Here's how the part is built. I have some questions about the finished solid (model axes, mm). Face numbers are marked on the shaded views. A direction names the side the tool comes from. Round coordinates to 2 decimals unless told otherwise and drop trailing zeros. Loops run counter-clockwise (first coordinate to the right, second up) from the corner with the lowest first, then second, coordinate; pieces in that order, holes last. Notation, with made-up numbers: (73.5, 27) - (88.5, 27) arc R13 ccw to (88.5, 41) - close; hole circle Ø11 at (-4, 51). An arc over 180 degrees is marked (long way). Answer as a JSON object with one key per item and string values. Group by question number.
1) Which directions (+Z, -Z, +X, -X, +Y, -Y) give clear straight access to the entire face, cutting with the end or side of a thin tool? Please do the marked faces 1, 2 and 3.
2) I want a section at A-A, the plane x = 3. Please give me the cut outline in (y, z).
3) Will these pins go through, and if not, where does the flat tip stop? P1, Ø4, axis at y = 22.5, z = 5.5, coming from the +X side; P2, Ø2, axis at y = 5, z = -2.5, coming from the -X side; P3, Ø3, axis at x = 18, z = -0.5, coming from the +Y side.
4) I want a section at B-B, the plane y = 33. Please give me the cut outline in (x, z), then the cut area to 3 significant figures.
5) If I drill on line 1 along X through (y, z) = (36, -5); line 2 along Y through (x, z) = (21, 5.5); line 3 along Y through (x, z) = (18, 1.75), over which ranges is the centre line in solid material (lowest first)? Write a range as [from, to].
from build123d import *

# Parameters (mm, degrees)
SKETCH_1_W             = 40
SKETCH_1_H             = 20
EXTRUDE_1_DEPTH        = 37
SKETCH_2_W             = 20
SKETCH_2_H             = 2.5
EXTRUDE_2_DEPTH        = 7
FILLET_1_R             = 1
CUT_EXTRUDE_1_DEPTH    = 47
FILLET_1_OF_MIRROR_1_R = 1
EXTRUDE_3_DEPTH        = 2.5
SKETCH_6_R             = 6.5
EXTRUDE_4_DEPTH        = 3.5
SKETCH_7_R             = 5.5
EXTRUDE_5_DEPTH        = 4
SKETCH_8_R             = 3
EXTRUDE_6_DEPTH        = 8
CHAMFER_1_SIZE         = 2


with BuildPart() as part:
    # 草图1 → 凸台-拉伸1 (new body)
    with BuildSketch(Plane(origin=(0, 0, 0), x_dir=(1, 0, 0), z_dir=(0, 1, 0))):
        Rectangle(SKETCH_1_W, SKETCH_1_H)
    extrude(amount=EXTRUDE_1_DEPTH)

    # 草图2 → 凸台-拉伸2 (add)
    with BuildSketch(Plane(origin=(20, 0, 0), x_dir=(0, 0, -1), z_dir=(1, 0, 0))):
        with Locations((0, 28.75)):
            Rectangle(SKETCH_2_W, SKETCH_2_H)
    extrude_2 = extrude(amount=EXTRUDE_2_DEPTH)

    # 圆角1
    fillet_1_edges = [part.edges().sort_by_distance(p)[0] for p in [
        (27, 28.75, -10),
        (27, 28.75, 10),
    ]]
    fillet(fillet_1_edges, radius=FILLET_1_R)

    # 草图3 → 切除-拉伸1 (cut)
    with BuildSketch(Plane(origin=(0, 0, 0), x_dir=(1, 0, 0), z_dir=(0, 1, 0))):
        with BuildLine():
            Line((25.882021082, 5.209730705), (27, 5.209730705))
            Line((27, 5.209730705), (27, 3.27640675))
            Line((27, 3.27640675), (25.792986763, 3.27640675))
            ThreePointArc((25.792986763, 3.27640675), (22.077686149, 4.416217577), (25.882021082, 5.209730705))
        make_face()
        with BuildLine():
            Line((27, -3.27640675), (25.792986763, -3.27640675))
            ThreePointArc((25.792986763, -3.27640675), (22.077686149, -4.416217577), (25.882021082, -5.209730705))
            Line((25.882021082, -5.209730705), (27, -5.209730705))
            Line((27, -5.209730705), (27, -3.27640675))
        make_face()
    cut_extrude_1 = extrude(amount=CUT_EXTRUDE_1_DEPTH, mode=Mode.SUBTRACT)

    # 镜向1: 凸台-拉伸2, 切除-拉伸1 across plane
    add(extrude_2.mirror(Plane(origin=(0, 0, 0), x_dir=(0, 0, 1), z_dir=(1, 0, 0))))
    add(cut_extrude_1.mirror(Plane(origin=(0, 0, 0), x_dir=(0, 0, 1), z_dir=(1, 0, 0))), mode=Mode.SUBTRACT)

    # 圆角1 of 镜向1
    fillet_1_of_mirror_1_edges = [part.edges().sort_by_distance(p)[0] for p in [
        (-27, 28.75, -10),
        (-27, 28.75, 10),
    ]]
    fillet(fillet_1_of_mirror_1_edges, radius=FILLET_1_OF_MIRROR_1_R)

    # 草图4 → 凸台-拉伸3 (add)
    with BuildSketch(Plane(origin=(0, 37, 0), x_dir=(1, 0, 0), z_dir=(0, 1, 0))):
        with BuildLine():
            Line((14, 10), (14, 3.303949568))
            ThreePointArc((14, 3.303949568), (15.996871366, 0), (14, -3.303949568))
            Line((14, -3.303949568), (14, -10))
            Line((14, -10), (-10, -10))
            ThreePointArc((-10, -10), (-20, 0), (-10, 10))
            Line((-10, 10), (14, 10))
        make_face()
    extrude(amount=EXTRUDE_3_DEPTH)

    # 草图6 → 凸台-拉伸4 (add)
    with BuildSketch(Plane(origin=(0, 37, 0), x_dir=(1, 0, 0), z_dir=(0, 1, 0))):
        with Locations(Location((-10, 0, 0), (0, 0, 270))):
            Circle(SKETCH_6_R)
    extrude(amount=EXTRUDE_4_DEPTH)

    # 草图7 → 凸台-拉伸5 (add)
    with BuildSketch(Plane(origin=(0, 37, 0), x_dir=(1, 0, 0), z_dir=(0, 1, 0))):
        with Locations(Location((-10, 0, 0), (0, 0, 270))):
            Circle(SKETCH_7_R)
    extrude(amount=EXTRUDE_5_DEPTH)

    # 草图8 → 凸台-拉伸6 (add)
    with BuildSketch(Plane(origin=(0, 37, 0), x_dir=(1, 0, 0), z_dir=(0, 1, 0))):
        with Locations(Location((-10, 0, 0), (0, 0, 270))):
            Circle(SKETCH_8_R)
    extrude(amount=EXTRUDE_6_DEPTH)

    # 倒角1
    chamfer_1_edges = [part.edges().sort_by_distance(p)[0] for p in [
        (0, 0, 10),
        (-20, 0, 0),
        (0, 0, -10),
        (20, 0, 0),
    ]]
    chamfer(chamfer_1_edges, length=CHAMFER_1_SIZE)


solid = part.part
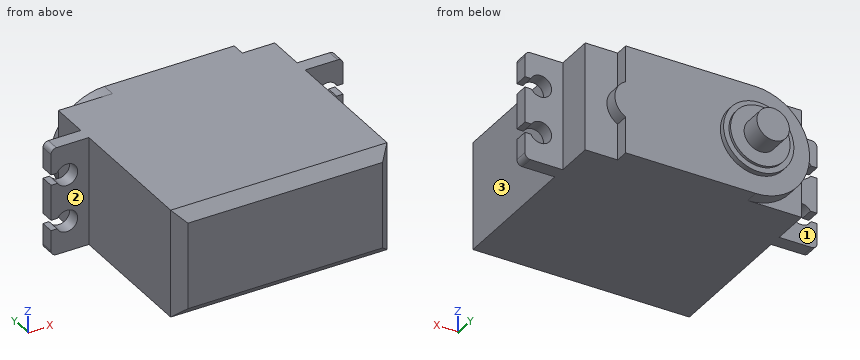
Outcome:
{
 "1": {"face 1": "+Z, -Z, -X, +Y", "face 2": "+Z, -Z, -X, -Y", "face 3": "+Z, -Z, +X, -Y"},
 "2": {"outline": "(0, -8) - (2, -10) - (39.5, -10) - (39.5, 10) - (2, 10) - (0, 8) - close"},
 "3": {"P1": "x = 20", "P2": "x = -20", "P3": "y = 37"},
 "4": {"outline": "(-20, -10) - (20, -10) - (20, 10) - (-20, 10) - close", "area": "800 mm^2"},
 "5": {"line 1": "[-20, 20]", "line 2": "[27.5, 30]", "line 3": "[0, 37]"}
}
